Can you work these out from the model? Positions are in its coordinate system, mm. A direction names the side the tool comes from. Give positions to 0.01 mm unless a question says otherwise; leave off trailing zeros. Loops run counter-clockwise (first coordinate to the right, second up) from the corner with the lowest first, then second, coordinate; pieces in that order, holes last. Notation, with made-up numbers: (23, 45) -> (60, 45) arc R14 ccw to (60, 61) -> close; hole circle Ø10 at (-11, 41.5). An arc over 180 degrees is marked (long way). One line per question, with ' | ' between items.
from build123d import *

# Parameters (mm, degrees)
SKETCH1_W            = 22
SKETCH1_H            = 60
SKETCH1_R            = 2.5
SKETCH1_W_2          = 4
BOSS_EXTRUDE1_DEPTH  = 15
SKETCH1_3_W          = 4
SKETCH1_3_H          = 60
BOSS_EXTRUDE2_DEPTH  = 40
M5_CLEARANCE_HOLE1_D = 5.3
LPATTERN1_COUNT      = 2
LPATTERN1_PITCH      = 20
FILLET1_R            = 1


with BuildPart() as part:
    # Sketch1 → Boss-Extrude1 (new body)
    # profile 1 of 3: a face of its own
    with BuildSketch(Plane(origin=(0, 0, 0), x_dir=(1, 0, 0), z_dir=(0, 1, 0))):
        Rectangle(SKETCH1_W, SKETCH1_H)
        with Locations(Location((0, -10, 0), (0, 0, 270))):
            Circle(SKETCH1_R, mode=Mode.SUBTRACT)
        with Locations(Location((0, 10, 0), (0, 0, 270))):
            Circle(SKETCH1_R, mode=Mode.SUBTRACT)
    # profile 2 of 3: a face of its own
    with BuildSketch(Plane(origin=(0, 0, 0), x_dir=(1, 0, 0), z_dir=(0, 1, 0))):
        with Locations((-13, 0)):
            Rectangle(SKETCH1_W_2, SKETCH1_H)
    # profile 3 of 3: a face of its own
    with BuildSketch(Plane(origin=(0, 0, 0), x_dir=(1, 0, 0), z_dir=(0, 1, 0))):
        with Locations((13, 0)):
            Rectangle(SKETCH1_W_2, SKETCH1_H)
    extrude(amount=-BOSS_EXTRUDE1_DEPTH)

    # Sketch1_3 → Boss-Extrude2 (add)
    with BuildSketch(Plane(origin=(0, 0, 0), x_dir=(1, 0, 0), z_dir=(0, 1, 0))):
        with Locations((-13, 0)):
            Rectangle(SKETCH1_3_W, SKETCH1_3_H)
        with Locations((13, 0)):
            Rectangle(SKETCH1_3_W, SKETCH1_3_H)
    extrude(amount=BOSS_EXTRUDE2_DEPTH)

    # M5 Clearance Hole1 (through all)
    with Locations(Plane(origin=(15, 10, 10), x_dir=(0, 0, 1), z_dir=(1, 0, 0))):
        with Locations((0, 0), (-20, 0)):
            m5_clearance_hole1 = Hole(M5_CLEARANCE_HOLE1_D / 2)

    # LPattern1: M5 Clearance Hole1 ×2
    with Locations(*[(0, i * LPATTERN1_PITCH, 0) for i in range(1, LPATTERN1_COUNT)]):
        add(m5_clearance_hole1, mode=Mode.SUBTRACT)

    # Fillet1
    fillet1_edges = [part.edges().sort_by_distance(p)[0] for p in [
        (-15, 12.5, 30),
        (-15, 12.5, -30),
        (15, 12.5, -30),
        (15, 12.5, 30),
        (-13, 40, -30),
        (-13, 40, 30),
        (13, 40, -30),
        (13, 40, 30),
    ]]
    fillet(fillet1_edges, radius=FILLET1_R)


solid = part.part
Q1. For pin 1 Ø11 at (x, z) = (-5, -3) entering from +Y; pin 2 Ø8.5 at (y, z) = (30, -10) entering from +X, each with a flat end and sliding along its axis, tell me the tip position at first contact or that it passes through.
Entries:
pin 1: y = 0 | pin 2: x = 15
Q2. If we mould it in two halves opening along X, with no side actions, what happens to faces 1 (the face through (13, 40, 0)), 2 (the face through (11, 20, 0)), 3 (the face through (15, 13, 0)), 4 (the face through (0.1, -7.4, -12.5))? For each: pulls with the +X half, pulls with the -X half, needs draft (parallel to the pull), parting line crosses it, or undercut.
Entries:
face 1: needs draft | face 2: undercut | face 3: pulls with the +X half | face 4: undercut
Q3. On a 3-axis mill with a long thin cutter (end or side, diameter ignored), from which of +Z, -Z, +X, -X, +Y, -Y can I reach the whole of each face in a straight line? I mean faces 5 (the face through (-13.03, 27.37, 10.34)), 6 (the face through (-11, 20, 0)). Say none if no direction works.
Entries:
face 5: +X, -X | face 6: +Z, -Z, +Y
Q4. If we section it at B-B (z = 10): Write out the boundary of the cut face in (x, y), plus the area to 3 significant figures.
Entries:
outline: (-15, -15) -> (-2.5, -15) -> (-2.5, 0) -> (-11, 0) -> (-11, 7.35) -> (-15, 7.35) -> close; (-15, 12.65) -> (-11, 12.65) -> (-11, 27.35) -> (-15, 27.35) -> close; (-15, 32.65) -> (-11, 32.65) -> (-11, 40) -> (-15, 40) -> close; (2.5, -15) -> (15, -15) -> (15, 7.35) -> (11, 7.35) -> (11, 0) -> (2.5, 0) -> close; (11, 12.65) -> (15, 12.65) -> (15, 27.35) -> (11, 27.35) -> close; (11, 32.65) -> (15, 32.65) -> (15, 40) -> (11, 40) -> close | area: 610 mm²
Q5. If we section it at A-A (y = 10): Write out the boundary of the cut face in (x, z), plus the area to 3 significant figures.
Entries:
outline: (-15, -29) arc R1 ccw to (-14, -30) -> (-11, -30) -> (-11, -12.65) -> (-15, -12.65) -> close; (-15, -7.35) -> (-11, -7.35) -> (-11, 7.35) -> (-15, 7.35) -> close; (-15, 12.65) -> (-11, 12.65) -> (-11, 30) -> (-14, 30) arc R1 ccw to (-15, 29) -> close; (11, -30) -> (14, -30) arc R1 ccw to (15, -29) -> (15, -12.65) -> (11, -12.65) -> close; (11, -7.35) -> (15, -7.35) -> (15, 7.35) -> (11, 7.35) -> close; (11, 12.65) -> (15, 12.65) -> (15, 29) arc R1 ccw to (14, 30) -> (11, 30) -> close | area: 394 mm²
Q6. If we section it at C-C (x = 0): Write out the boundary of the cut face in (y, z), plus the area to 3 significant figures.
Entries:
outline: (-15, -30) -> (0, -30) -> (0, -12.5) -> (-15, -12.5) -> close; (-15, -7.5) -> (0, -7.5) -> (0, 7.5) -> (-15, 7.5) -> close; (-15, 12.5) -> (0, 12.5) -> (0, 30) -> (-15, 30) -> close | area: 750 mm²
Q7. If we section it at D-D (y = 4.5): Write out the boundary of the cut face in (x, z), plus the area to 3 significant figures.
Entries:
outline: (-15, -29) arc R1 ccw to (-14, -30) -> (-11, -30) -> (-11, 30) -> (-14, 30) arc R1 ccw to (-15, 29) -> close; (11, -30) -> (14, -30) arc R1 ccw to (15, -29) -> (15, 29) arc R1 ccw to (14, 30) -> (11, 30) -> close | area: 479 mm²
Q8. If I drill on probe 1 along Z at (x, y) = (-12.6, 30); probe 2 along Y at (x, z) = (-12.7, 10); probe 3 along X at (y, z) = (8.5, -5.5), over which ranges is the centre line in solid material (lowest first)? Write a range as from..to.
Entries:
probe 1: -30..-12.65, -7.35..7.35, 12.65..30 | probe 2: -15..7.35, 12.65..27.35, 32.65..40 | probe 3: -15..-11, 11..15
